```python
from build123d import *

# Parameters (mm, degrees)
BOSS_EXTRUDE1_DEPTH = 10
CHAMFER1_SIZE       = 2
SKETCH2_R           = 1.75
CUT_EXTRUDE1_DEPTH  = 11
LPATTERN1_COUNT     = 5
LPATTERN1_PITCH     = 10
SKETCH3_R           = 1.5
CUT_EXTRUDE2_DEPTH  = 10


with BuildPart() as part:
    # Sketch1 → Boss-Extrude1 (new body)
    with BuildSketch(Plane.XY):
        with BuildLine():
            Line((-106, 0), (-106, 60))
            ThreePointArc((-106, 60), (0, 166), (106, 60))
            Line((106, 60), (106, 0))
            Line((106, 0), (96, 0))
            Line((96, 0), (96, 60))
            ThreePointArc((96, 60), (0, 156), (-96, 60))
            Line((-96, 60), (-96, 0))
            Line((-96, 0), (-106, 0))
        make_face()
    extrude(amount=BOSS_EXTRUDE1_DEPTH)

    # Chamfer1
    chamfer1_edges = [part.edges().sort_by_distance(p)[0] for p in [
        (96, 30, 0),
        (0, 156, 0),
        (-96, 30, 0),
        (0, 156, 10),
        (96, 30, 10),
        (106, 30, 10),
        (0, 166, 10),
        (-106, 30, 10),
        (-106, 30, 0),
        (-96, 30, 10),
        (0, 166, 0),
        (106, 30, 0),
    ]]
    chamfer(chamfer1_edges, length=CHAMFER1_SIZE)

    # Sketch2 → Cut-Extrude1 (cut, through all)
    with BuildSketch(Plane.XY.offset(10)):
        with Locations((-101, 12.5)):
            Circle(SKETCH2_R)
        with Locations((101, 12.5)):
            Circle(SKETCH2_R)
    cut_extrude1 = extrude(amount=-CUT_EXTRUDE1_DEPTH, mode=Mode.SUBTRACT)

    # LPattern1: Cut-Extrude1 ×5
    with Locations(*[(0, i * LPATTERN1_PITCH, 0) for i in range(1, LPATTERN1_COUNT)]):
        add(cut_extrude1, mode=Mode.SUBTRACT)

    # Sketch3 → Cut-Extrude2 (cut)
    with BuildSketch(Plane.XZ):
        with Locations((-101, 5)):
            Circle(SKETCH3_R)
        with Locations((101, 5)):
            Circle(SKETCH3_R)
    extrude(amount=-CUT_EXTRUDE2_DEPTH, mode=Mode.SUBTRACT)


solid = part.part
```
Could you check a few things on this model? Use its own coordinates, in mm. A direction names the side the tool comes from. Round coordinates to 2 decimals unless told otherwise and drop trailing zeros. Write each loop counter-clockwise with the first axis right and the second up, starting at its lowest first coordinate (ties: lowest second). Pieces come first, ordered by that corner, then holes.
(1) If I drill on probe 1 along Z at (x, y) = (-101, 5.5); probe 2 along X at (y, z) = (53.5, 9.75); probe 3 along X at (y, z) = (20, 2), over which ranges is the centre line in solid material (lowest first)?
Findings below:
probe 1: z = 0 to 3.5, 6.5 to 10
probe 2: x = -104.25 to -102.44, -99.56 to -97.75, 97.75 to 99.56, 102.44 to 104.25
probe 3: x = -106 to -96, 96 to 106
(2) Thinking about a two-plate mould opening in X: for faces 3 (the face through (106, 30, 5)), 4 (the face through (2.111, 155.977, 4.958)), 5 (the face through (-2.294, 164.294, 0.319)), 6 (the face through (-30, 155, 0)), which applies, +X half, -X half, draft (parallel to the pull), parting line (faces both ways), or undercut?
Findings below:
face 3: +X half
face 4: undercut
face 5: parting line
face 6: draft
(3) Which directions (+Z, -Z, +X, -X, +Y, -Y) give clear straight access to the entire face, cutting with the end or side of a thin tool? Please do faces 1 (the face through (-2.294, 164.294, 9.681)), 2 (the face through (-96, 30, 5)).
Findings below:
face 1: +Z, +Y
face 2: +Z, -Z, -Y
(4) Suppose I cut it at A-A on x = 0. Write out the boundary of the cut face in (y, z), and give its area (3 significant figures).
Findings below:
outline: (156, 2) - (158, 0) - (164, 0) - (166, 2) - (166, 8) - (164, 10) - (158, 10) - (156, 8) - close
area: 92.0 mm2
(5) For pin 1 (4 mm diameter, centred on x = -67, z = 2, fed in from -Y); pin 2 (3 mm diameter, centred on y = 68.5, z = 7.5, fed in from -X); pin 3 (2 mm diameter, centred on x = -77.5, z = 4.5, fed in from +Y), each with a flat end and sliding along its axis, tell me the tip position at first contact or that it passes through.
Findings below:
pin 1: stops at y = 126.75
pin 2: stops at x = -105.77
pin 3: stops at y = 133.37
